Build history of the part. All positions in model axes, mm. A direction names the side the tool comes from. Coordinates: 2 decimals unless noted, no trailing zeros. Write each loop counter-clockwise with the first axis right and the second up, starting at its lowest first coordinate (ties: lowest second). Pieces come first, ordered by that corner, then holes. Notation, with made-up numbers: (-16.75, 80.5) -> (-12.75, 80.5) arc R12 ccw to (-12.75, 97.5) -> close; hole circle Ø4 at (18, 31.5). An arc over 180 degrees is marked (long way). Write each question's results on one line, items separated by ' | '. Start each with the question number.
Q1. Tool access for faces 4 (the face through (-19.213, -7.056, -7.516)), 5 (the face through (23, -7, 4.289)), 6 (the face through (2, -7, -15.711)): list every direction of +Z, -Z, +X, -X, +Y, -Y with a clear straight run to the whole face (end or side of a thin tool).
Q2. Saw through at D-D on y = -1. Give the cut face in (x, z), and give its area (3 significant figures).
Q3. Drill centre lines: line 1 (X direction, y = -10.75, z = -2); line 2 (Z direction, x = 26, y = -4); line 3 (X direction, y = -0.25, z = 16). Where is each one in solid material? Low to high.
Q4. Saw through at B-B on z = 1. Give the cut face in (x, y).
Q5. Saw through at C-C on x = -17. Give the cut face in (y, z).
Q6. Saw through at A-A on y = -8.5. Give the cut face in (x, z), and give its area (3 significant figures).
Q7. Two-plate mould, pull along Y, no slides. Class faces 1 (the face through (28.857, -7, -6)), 2 (the face through (2, -15, -2)), 3 (the face through (16.357, -7.387, 11.387)): released by +Y, released by -Y, zero draft, split by the parting line, or undercut.
from build123d import *

# Parameters (mm, degrees)
F0_W     = 53
F0_H     = 34
F1_DEPTH = 15
F2_R     = 27
F3_DEPTH = 10
F5_DEPTH = 14


with BuildPart() as f1:
    # F0 (on Front) → F1 (new body)
    with BuildSketch(Plane.XZ):
        with Locations((2.3567589563, 1.288594678)):
            Rectangle(F0_W, F0_H)
    extrude(amount=F1_DEPTH)

    # F2 (on face) → F3 (cut)
    with BuildSketch(Plane(origin=(-24.1432410437, 0, 0), x_dir=(0, -1, 0), z_dir=(-1, 0, 0))):
        with Locations((15, 18.288594678)):
            Circle(F2_R)
    extrude(amount=-F3_DEPTH, mode=Mode.SUBTRACT)

    # F4 (on face) → F5 (cut)
    with BuildSketch(Plane.XY.offset(18.288594678)):
        with BuildLine():
            Line((28.8567589563, 0), (18.8567589563, 0))
            ThreePointArc((18.8567589563, 0), (16.3567589563, -7.5), (18.8567589563, -15))
            Line((18.8567589563, -15), (28.8567589563, -15))
            Line((28.8567589563, -15), (28.8567589563, 0))
        make_face()
    extrude(amount=-F5_DEPTH, mode=Mode.SUBTRACT)


solid = f1.part
Returned:
1) face 4: +Z, -X, -Y | face 5: +Z, +X | face 6: -Z, +X, -X, +Y, -Y
2) outline: (-24.14, -15.71) -> (28.86, -15.71) -> (28.86, 4.29) -> (18.18, 4.29) -> (18.18, 18.29) -> (-14.14, 18.29) -> (-14.14, -4.8) -> (-24.14, -4.8) -> close | area: 1,420 mm2
3) line 1: x = -14.14 to 28.86 | line 2: z = -15.71 to 4.29 | line 3: x = -14.14 to 18.67
4) outline: (-14.14, -15) -> (28.86, -15) -> (28.86, 0) -> (-14.14, 0) -> close
5) outline: (-15, -15.71) -> (0, -15.71) -> (0, -4.16) arc R27 cw to (-15, -8.71) -> close
6) outline: (-24.14, -15.71) -> (28.86, -15.71) -> (28.86, 4.29) -> (16.4, 4.29) -> (16.4, 18.29) -> (-14.14, 18.29) -> (-14.14, -7.92) -> (-24.14, -7.92) -> close | area: 1,370 mm2
7) face 1: zero draft | face 2: released by -Y | face 3: undercut
